Work out the finished part from the listing and answer in its coordinate system (mm). Coordinates: 2 decimals unless noted, no trailing zeros. Write each loop counter-clockwise with the first axis right and the second up, starting at its lowest first coordinate (ties: lowest second). Pieces come first, ordered by that corner, then holes. Notation, with made-up numbers: (-23, 68) - (22, 68) arc R27 cw to (22, 98) - close; hole circle Ø11 at (80.5, 25.25). An arc over 180 degrees is marked (long way). Use CSV: the item, a comma, the result in double quotes. Start each with the question number.
from build123d import *

# Parameters (mm, degrees)
SKETCH4_R           = 29
SKETCH4_R_2         = 26
BOSS_EXTRUDE1_DEPTH = 2380
CUT_EXTRUDE1_DEPTH  = 2381.883239472
FILLET1_R           = 1


with BuildPart() as part:
    # Sketch4 → Boss-Extrude1 (new body)
    with BuildSketch(Plane.XY):
        with Locations((29, 0)):
            Circle(SKETCH4_R)
        with Locations((29, 0)):
            Circle(SKETCH4_R_2, mode=Mode.SUBTRACT)
    extrude(amount=-BOSS_EXTRUDE1_DEPTH)

    # Sketch6 → Cut-Extrude1 (cut, through all)
    with BuildSketch(Plane(origin=(0, 0, 0), x_dir=(0, 0, -1), z_dir=(1, 0, 0))):
        with BuildLine():
            Line((0, 10), (0, -10))
            Line((0, -10), (15, -10))
            ThreePointArc((15, -10), (25, 0), (15, 10))
            Line((15, 10), (0, 10))
        make_face()
    extrude(amount=CUT_EXTRUDE1_DEPTH, mode=Mode.SUBTRACT)

    # Fillet1
    fillet1_edges = [part.edges().sort_by_distance(p)[0] for p in [
        (3.389342411, 10, 0),
        (54.610657589, 10, 0),
        (3.389342411, -10, 0),
        (54.610657589, -10, 0),
    ]]
    fillet(fillet1_edges, radius=FILLET1_R)


solid = part.part
Item 1: Each of these flat-tipped pins is pushed along its axis until it touches: pin 1 (5 mm diameter, centred on y = -17, z = -1609.5, fed in from +X); pin 2 (3 mm diameter, centred on x = 36.5, z = -291, fed in from +Y); pin 3 (1.6 mm diameter, centred on x = 3.5, z = -10.5, fed in from +Y). Where does it stop, or does it pass through?
Item 2: Straight lines are drawn through the part: probe 1 along Y at (x, z) = (29, -864); probe 2 along X at (y, z) = (-10, -873); probe 3 along X at (y, z) = (0, -740.5). For each, find the intervals that lie inside material, in ascending order. Write a range as [from, to].
Item 3: A cutting plane is placed at C-C (z = -926.5). Determine the outline of the cut face in (x, y).
Item 4: A cutting plane is placed at B-B (y = 0). Determine the outline of the cut face in (x, z).
Item 5: A cutting plane is placed at A-A (x = 29). Determine the outline of the cut face in (y, z), then the cut area to 3 significant figures.
Item 6: Determine the mould class of faces 1 (the face through (53.8, 7.81, -1173.34)), 2 (the face through (5.99, -17.65, -1173.34)), 3 (the face through (18, 24, -2380)) for opening direction X: +X half, -X half, draft (parallel to the pull), parting line (faces both ways), or undercut.
Calculated:
1,pin 1,"stops at x = 54.11"
1,pin 2,"stops at y = 28.37"
1,pin 3,"stops at y = 15.2"
2,probe 1,"y = [-29, -26], [26, 29]"
2,probe 2,"x = [1.78, 5], [53, 56.22]"
2,probe 3,"x = [0, 3], [55, 58]"
3,outline,"circle Ø58 at (29, 0); hole circle Ø52 at (29, 0)"
4,outline,"(0, -2380) - (3, -2380) - (3, -25) - (0, -25) - close; (55, -2380) - (58, -2380) - (58, -25) - (55, -25) - close"
5,outline,"(-29, -2380) - (-26, -2380) - (-26, 0) - (-29, 0) - close; (26, -2380) - (29, -2380) - (29, 0) - (26, 0) - close"
5,area,"14,300 mm²"
6,face 1,"undercut"
6,face 2,"parting line"
6,face 3,"draft"
